from build123d import *

# Parameters (mm, degrees)
F0_W     = 329.6
F0_H     = 521.4
F0_R     = 18
F0_W_2   = 6
F0_H_2   = 25
F0_R_2   = 12.5
F1_DEPTH = 6
F2_W     = 6
F2_H     = 92.85
F2_H_2   = 50
F3_DEPTH = 25
F5_W     = 25
F5_H     = 6
F6_DEPTH = 25
F7_DEPTH = 25


with BuildPart() as f1:
    # F0 (on Top) → F1 (new body)
    with BuildSketch(Plane.XY):
        with Locations((0, 234.753206)):
            Rectangle(F0_W, F0_H)
        with Locations((-82.4, 234.753206)):
            Circle(F0_R, mode=Mode.SUBTRACT)
        with Locations((-42.8, 326.553206)):
            Rectangle(F0_W_2, F0_H_2, mode=Mode.SUBTRACT)
        with Locations((-42.8, 391.553206)):
            Rectangle(F0_W_2, F0_H_2, mode=Mode.SUBTRACT)
        with Locations((0, 234.753206)):
            Circle(F0_R_2, mode=Mode.SUBTRACT)
        with Locations((34.2, 326.553206)):
            Rectangle(F0_W_2, F0_H_2, mode=Mode.SUBTRACT)
        with Locations((82.4, 234.753206)):
            Circle(F0_R, mode=Mode.SUBTRACT)
        with Locations((34.2, 391.553206)):
            Rectangle(F0_W_2, F0_H_2, mode=Mode.SUBTRACT)
    extrude(amount=F1_DEPTH)

    # F2 (on face) → F3 (cut)
    with BuildSketch(Plane.XY.offset(6)):
        with Locations((-161.8, 449.028206)):
            Rectangle(F2_W, F2_H)
        with Locations((-161.8, 331.178206)):
            Rectangle(F2_W, F2_H)
        with Locations((-161.8, 234.753206)):
            Rectangle(F2_W, F2_H_2)
        with Locations((-161.8, 138.328206)):
            Rectangle(F2_W, F2_H)
        with Locations((-161.8, 20.478206)):
            Rectangle(F2_W, F2_H)
        with Locations((161.8, 449.028206)):
            Rectangle(F2_W, F2_H)
        with Locations((161.8, 20.478206)):
            Rectangle(F2_W, F2_H)
        with Locations((161.8, 138.328206)):
            Rectangle(F2_W, F2_H)
        with Locations((161.8, 331.178206)):
            Rectangle(F2_W, F2_H)
        with Locations((161.8, 234.753206)):
            Rectangle(F2_W, F2_H_2)
    extrude(amount=-F3_DEPTH, mode=Mode.SUBTRACT)

    # F5 (on face) → F6 (cut)
    with BuildSketch(Plane.XY.offset(6)):
        with Locations((-64.8, 317.053206)):
            Rectangle(F5_W, F5_H)
        with Locations((-64.8, 401.053206)):
            Rectangle(F5_W, F5_H)
        with Locations((56.2, 401.053206)):
            Rectangle(F5_W, F5_H)
        with Locations((56.2, 317.053206)):
            Rectangle(F5_W, F5_H)
        with BuildLine():
            Line((3.2, 421.553206), (-11.8, 421.553206))
            ThreePointArc((-11.8, 421.553206), (-15.335534, 420.08874), (-16.8, 416.553206))
            Line((-16.8, 416.553206), (-16.8, 301.553206))
            ThreePointArc((-16.8, 301.553206), (-15.335534, 298.017672), (-11.8, 296.553206))
            Line((-11.8, 296.553206), (3.2, 296.553206))
            ThreePointArc((3.2, 296.553206), (6.735534, 298.017672), (8.2, 301.553206))
            Line((8.2, 301.553206), (8.2, 416.553206))
            ThreePointArc((8.2, 416.553206), (6.735534, 420.08874), (3.2, 421.553206))
        make_face()
    extrude(amount=-F6_DEPTH, mode=Mode.SUBTRACT)

    # F4 (on face) → F7 (cut)
    with BuildSketch(Plane.XY.offset(6)):
        with BuildLine():
            Line((54.8, 166.053206), (-79.8, 166.053206))
            ThreePointArc((-79.8, 166.053206), (-82.628427, 164.881633), (-83.8, 162.053206))
            Line((-83.8, 162.053206), (-83.8, 160.053206))
            ThreePointArc((-83.8, 160.053206), (-82.628427, 157.224779), (-79.8, 156.053206))
            Line((-79.8, 156.053206), (54.8, 156.053206))
            ThreePointArc((54.8, 156.053206), (57.628427, 157.224779), (58.8, 160.053206))
            Line((58.8, 160.053206), (58.8, 162.053206))
            ThreePointArc((58.8, 162.053206), (57.628427, 164.881633), (54.8, 166.053206))
        make_face()
        with BuildLine():
            Line((54.8, 4.053206), (-79.8, 4.053206))
            ThreePointArc((-79.8, 4.053206), (-82.628427, 2.881633), (-83.8, 0.053206))
            Line((-83.8, 0.053206), (-83.8, -1.946794))
            ThreePointArc((-83.8, -1.946794), (-82.628427, -4.775221), (-79.8, -5.946794))
            Line((-79.8, -5.946794), (54.8, -5.946794))
            ThreePointArc((54.8, -5.946794), (57.628427, -4.775221), (58.8, -1.946794))
            Line((58.8, -1.946794), (58.8, 0.053206))
            ThreePointArc((58.8, 0.053206), (57.628427, 2.881633), (54.8, 4.053206))
        make_face()
    extrude(amount=-F7_DEPTH, mode=Mode.SUBTRACT)


solid = f1.part
Part model, mm, in its own coordinate system. Give positions to 0.01 mm unless a question says otherwise; leave off trailing zeros. Loops run counter-clockwise (first coordinate to the right, second up) from the corner with the lowest first, then second, coordinate; pieces in that order, holes last.
(1) Pull direction X, two halves, no side cores. Call faces 1 (the flat face through (-39, 238, 6)), 2 (the cylindrical face through (92.08, 249.93, 2.96)): pulls with the +X half, pulls with the -X half, needs draft (parallel to the pull), parting line crosses it, or undercut.
Return value:
face 1: needs draft
face 2: undercut
(2) Band-saw the part on B-B (y = 327). Write the cut outline in (x, z).
Return value:
outline: (-158.8, 0) - (-45.8, 0) - (-45.8, 6) - (-158.8, 6) - close; (-39.8, 0) - (-16.8, 0) - (-16.8, 6) - (-39.8, 6) - close; (8.2, 0) - (31.2, 0) - (31.2, 6) - (8.2, 6) - close; (37.2, 0) - (158.8, 0) - (158.8, 6) - (37.2, 6) - close
(3) Pin check, flat tips, straight feed: pin 1 (3 mm diameter, centred on x = -160.5, z = 4, fed in from -Y); pin 2 (1 mm diameter, centred on y = 180, z = 2.5, fed in from -X); pin 3 (2 mm diameter, centred on y = 98, z = 2, fed in from +X). Stop position of each tip, or through.
Return value:
pin 1: stops at y = 66.9
pin 2: stops at x = -158.8
pin 3: stops at x = 158.8
(4) Band-saw the part on A-A (x = 82.4). Write the cut outline in (y, z), and give its area (3 significant figures).
Return value:
outline: (-25.95, 0) - (216.75, 0) - (216.75, 6) - (-25.95, 6) - close; (252.75, 0) - (495.45, 0) - (495.45, 6) - (252.75, 6) - close
area: 2,910 mm2
(5) Drill centre lines: line 1 along Y through (x, z) = (38.5, 3.4); line 2 along Y through (x, z) = (0, 2.8); line 3 along X through (y, z) = (400, 3.5). Where is each one in solid material? Low to high.
Return value:
line 1: y = -25.95 to -5.95, 4.05 to 156.05, 166.05 to 495.45
line 2: y = -25.95 to -5.95, 4.05 to 156.05, 166.05 to 222.25, 247.25 to 296.55, 421.55 to 495.45
line 3: x = -164.8 to -77.3, -52.3 to -45.8, -39.8 to -16.8, 8.2 to 31.2, 37.2 to 43.7, 68.7 to 164.8
(6) Band-saw the part on D-D (y = 453). Write the cut outline in (x, z).
Return value:
outline: (-158.8, 0) - (158.8, 0) - (158.8, 6) - (-158.8, 6) - close
(7) Band-saw the part on C-C (z = 5). Count the separate pieces of the cut face and the enclosed holes in it, and give its area (3 significant figures).
Return value:
separate pieces: 1
enclosed holes: 14
area: 157,000 mm2
